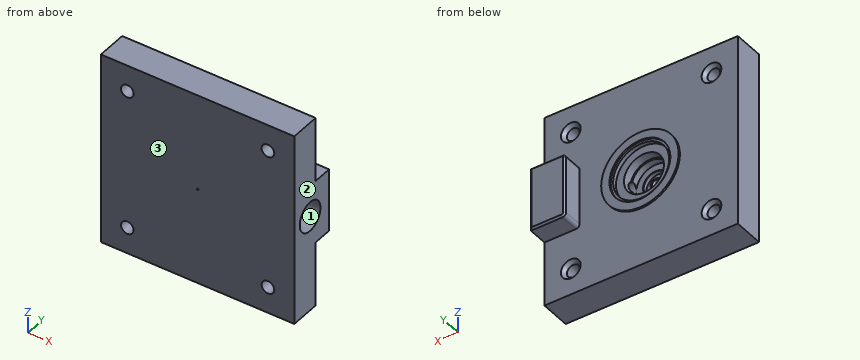
```python
from build123d import *

# Parameters (mm, degrees)
SKETCH2_W               = 55
SKETCH2_H               = 55
SKETCH2_R               = 20
BOSS_EXTRUDE1_DEPTH     = 8.6446
CUT_EXTRUDE1_REACH      = 63.947
CUT_EXTRUDE1_END_RADIUS = 5.47
SKETCH3_R               = 1.5
CUT_EXTRUDE2_REACH      = 41.84
SKETCH4_R               = 1.8
CHAMFER1_SIZE           = 1
BOSS_EXTRUDE2_DEPTH     = 6
SKETCH8_R               = 4.2164
CUT_EXTRUDE5_DEPTH      = 7
CHAMFER2_SIZE           = 0.5
CHAMFER3_SIZE           = 0.75


# Read off the part's stored shape, not the designer's step: Revolve2
with BuildPart() as part:
    # Revolve2 outline → Revolve2 (revolve)
    with BuildSketch(Plane.XY):
        Polygon((20, -7.4946), (20, 1.15), (11.01, 1.15), (11.01, 1.65), (8.65, 1.65), (8.65, 1.15), (7.97, 1.15), (7.97, 0), (5.681592205, 0), (5.681592205, -2.5658216), (5.47, -2.777413805), (5.47, -4.75), (3.57599, -4.75), (3.47599, -4.85), (3.47599, -5.9946), (1.52019, -5.9946), (1.52019, -4.85), (1.42019, -4.75), (0.25, -4.75), (0.25, -7.4946), align=None)
    revolve(axis=Axis((0, 0, 0), (0, 1, 0)))

    # Sketch2 → Boss-Extrude1 (add)
    with BuildSketch(Plane(origin=(0, 1.15, 0), x_dir=(1, 0, 0), z_dir=(0, 1, 0))):
        Rectangle(SKETCH2_W, SKETCH2_H)
        Circle(SKETCH2_R, mode=Mode.SUBTRACT)
    extrude(amount=-BOSS_EXTRUDE1_DEPTH)

    # Cut-Extrude1: up to this cylinder (the profile starts outside it)
    cut_extrude1_end = Plane(origin=(0, -3.2946, 0), z_dir=(0, 1, 0)) * Cylinder(CUT_EXTRUDE1_END_RADIUS, 139.834, mode=Mode.PRIVATE)
    # Sketch3 → Cut-Extrude1 (cut, up to the surface)
    with BuildSketch(Plane(origin=(27.5, 0, 0), x_dir=(0, 0, -1), z_dir=(1, 0, 0)), mode=Mode.PRIVATE) as cut_extrude1_sk1:
        with Locations((0, -3.2946)):
            Circle(SKETCH3_R)
    cut_extrude1_tool1 = extrude(cut_extrude1_sk1.sketch, amount=-CUT_EXTRUDE1_REACH, mode=Mode.PRIVATE) - cut_extrude1_end
    add(cut_extrude1_tool1.solids().sort_by_distance((27.5, -3.2946, 0))[0], mode=Mode.SUBTRACT)

    # Sketch4 → Cut-Extrude2 (cut, up to next)
    with BuildSketch(Plane(origin=(0, 1.15, 0), x_dir=(1, 0, 0), z_dir=(0, 1, 0)), mode=Mode.PRIVATE) as cut_extrude2_sk1:
        with Locations(Location((20, 20, 0), (0, 0, 180))):
            Circle(SKETCH4_R)
    cut_extrude2_tool1 = extrude(cut_extrude2_sk1.sketch, amount=-CUT_EXTRUDE2_REACH, mode=Mode.PRIVATE) & part.part
    # Sketch4 → Cut-Extrude2 (cut, up to next)
    with BuildSketch(Plane(origin=(0, 1.15, 0), x_dir=(1, 0, 0), z_dir=(0, 1, 0)), mode=Mode.PRIVATE) as cut_extrude2_sk2:
        with Locations(Location((20, -20, 0), (0, 0, 180))):
            Circle(SKETCH4_R)
    cut_extrude2_tool2 = extrude(cut_extrude2_sk2.sketch, amount=-CUT_EXTRUDE2_REACH, mode=Mode.PRIVATE) & part.part
    # Sketch4 → Cut-Extrude2 (cut, up to next)
    with BuildSketch(Plane(origin=(0, 1.15, 0), x_dir=(1, 0, 0), z_dir=(0, 1, 0)), mode=Mode.PRIVATE) as cut_extrude2_sk3:
        with Locations(Location((-20, -20, 0), (0, 0, 180))):
            Circle(SKETCH4_R)
    cut_extrude2_tool3 = extrude(cut_extrude2_sk3.sketch, amount=-CUT_EXTRUDE2_REACH, mode=Mode.PRIVATE) & part.part
    # Sketch4 → Cut-Extrude2 (cut, up to next)
    with BuildSketch(Plane(origin=(0, 1.15, 0), x_dir=(1, 0, 0), z_dir=(0, 1, 0)), mode=Mode.PRIVATE) as cut_extrude2_sk4:
        with Locations(Location((-20, 20, 0), (0, 0, 180))):
            Circle(SKETCH4_R)
    cut_extrude2_tool4 = extrude(cut_extrude2_sk4.sketch, amount=-CUT_EXTRUDE2_REACH, mode=Mode.PRIVATE) & part.part
    add(cut_extrude2_tool1.solids().sort_by_distance((20, 1.15, -20))[0], mode=Mode.SUBTRACT)
    add(cut_extrude2_tool2.solids().sort_by_distance((20, 1.15, 20))[0], mode=Mode.SUBTRACT)
    add(cut_extrude2_tool3.solids().sort_by_distance((-20, 1.15, 20))[0], mode=Mode.SUBTRACT)
    add(cut_extrude2_tool4.solids().sort_by_distance((-20, 1.15, -20))[0], mode=Mode.SUBTRACT)

    # Chamfer1
    chamfer1_edges = [part.edges().sort_by_distance(p)[0] for p in [
        (-18.2, 1.15, -20),
        (-18.2, 1.15, 20),
        (21.8, 1.15, 20),
        (21.8, 1.15, -20),
    ]]
    chamfer(chamfer1_edges, length=CHAMFER1_SIZE)

    # Sketch9 → Boss-Extrude2 (add)
    with BuildSketch(Plane(origin=(0, 1.15, 0), x_dir=(1, 0, 0), z_dir=(0, 1, 0))):
        with BuildLine():
            Line((18.5, 9), (27.5, 9))
            Line((27.5, 9), (27.5, -9))
            Line((27.5, -9), (18.5, -9))
            ThreePointArc((18.5, -9), (17.792893219, -8.707106781), (17.5, -8))
            Line((17.5, -8), (17.5, 8))
            ThreePointArc((17.5, 8), (17.792893219, 8.707106781), (18.5, 9))
        make_face()
    extrude(amount=BOSS_EXTRUDE2_DEPTH)

    # Sketch8 → Cut-Extrude5 (cut)
    with BuildSketch(Plane(origin=(27.5, 0, 0), x_dir=(0, 0, -1), z_dir=(1, 0, 0))):
        with Locations((0, -1.0782)):
            Circle(SKETCH8_R)
    extrude(amount=-CUT_EXTRUDE5_DEPTH, mode=Mode.SUBTRACT)

    # Chamfer2
    chamfer2_edges = [part.edges().sort_by_distance(p)[0] for p in [
        (27.5, 7.15, 0),
        (23, 7.15, -9),
        (17.792893219, 7.15, -8.707106781),
        (17.5, 7.15, 0),
        (17.792893219, 7.15, 8.707106781),
        (23, 7.15, 9),
    ]]
    chamfer(chamfer2_edges, length=CHAMFER2_SIZE)

    # Chamfer3
    chamfer3_edges = [part.edges().sort_by_distance(p)[0] for p in [
        (-0.25, -4.75, 0),
    ]]
    chamfer(chamfer3_edges, length=CHAMFER3_SIZE)


solid = part.part
```
Geometry: final body of the model. Coordinates: model frame, mm. Face numbers are marked on the shaded views. Give positions to 0.01 mm unless a question says otherwise; leave off trailing zeros. Loops run counter-clockwise (first coordinate to the right, second up) from the corner with the lowest first, then second, coordinate; pieces in that order, holes last. Notation, with made-up numbers: (-39.5, 63.5) -> (-10.5, 63.5) arc R26 cw to (-10.5, 96.5) -> close; hole circle Ø11 at (-2, 56). An arc over 180 degrees is marked (long way). Use one line per item in the form item = value.
Item 1: Section query A-A on z = 20. Output: boundary loops of the cut face in (x, y).
A:
outline = (-27.5, -7.49) -> (-21.8, -7.49) -> (-21.8, 0.15) -> (-22.8, 1.15) -> (-27.5, 1.15) -> close; (-18.2, -7.49) -> (18.2, -7.49) -> (18.2, 0.15) -> (17.2, 1.15) -> (-17.2, 1.15) -> (-18.2, 0.15) -> close; (21.8, -7.49) -> (27.5, -7.49) -> (27.5, 1.15) -> (22.8, 1.15) -> (21.8, 0.15) -> close
Item 2: Line query: probe 1 along X at (y, z) = (1.3, 0); probe 2 along Y at (x, z) = (14, 0); probe 3 along X at (y, z) = (0.75, 0). Output: solid intervals per line, ascending.
A:
probe_1 = -11.01 to -8.65, 8.65 to 11.01, 17.5 to 20.5
probe_2 = -7.49 to -4.79, -1.79 to 1.15
probe_3 = -27.5 to -7.97, 7.97 to 20.5
Item 3: Pin query (flat end, axial travel): P1, Ø1.4, axis at x = 0.5, z = 0.5, coming from the +Y side; P2, Ø1.5, axis at x = 4, z = -3.5, coming from the +Y side; P3, Ø18.5, axis at x = 0, z = 0, coming from the -Y side; P4, Ø2, axis at x = 5.5, z = 17, coming from the +Y side. Return the tip coordinate at first contact, or that it passes through.
A:
P1 = -4.75
P2 = 0
P3 = -7.49
P4 = 1.15
Item 4: Draft query along Y for the marked faces 1, 2 and 3. Return one class per face: pulls with the +Y half, pulls with the -Y half, needs draft (parallel to the pull), parting line crosses it, or undercut.
A:
face_1 = undercut
face_2 = needs draft
face_3 = pulls with the -Y half
Item 5: Section query D-D on x = -14. Output: boundary loops of the cut face in (y, z), and give its area (3 significant figures).
A:
outline = (-7.49, -27.5) -> (1.15, -27.5) -> (1.15, 27.5) -> (-7.49, 27.5) -> close
area = 475 mm^2
Item 6: Section query C-C on x = 23.5. Output: boundary loops of the cut face in (y, z), and give its area (3 significant figures).
A:
outline = (-7.49, -27.5) -> (1.15, -27.5) -> (1.15, -9) -> (6.65, -9) -> (7.15, -8.5) -> (7.15, 8.5) -> (6.65, 9) -> (1.15, 9) -> (1.15, 27.5) -> (-7.49, 27.5) -> close; hole circle Ø8.43 at (-1.08, 0)
area = 527 mm^2
Item 7: Section query B-B on x = -20. Output: boundary loops of the cut face in (y, z), and give its area (3 significant figures).
A:
outline = (-7.49, -27.5) -> (1.15, -27.5) -> (1.15, -22.8) -> (0.15, -21.8) -> (-7.49, -21.8) -> close; (-7.49, -18.2) -> (0.15, -18.2) -> (1.15, -17.2) -> (1.15, 17.2) -> (0.15, 18.2) -> (-7.49, 18.2) -> close; (-7.49, 21.8) -> (0.15, 21.8) -> (1.15, 22.8) -> (1.15, 27.5) -> (-7.49, 27.5) -> close
area = 411 mm^2
